The listing builds one solid part. Answer for the finished solid, in the listing's coordinates (mm). Face numbers are marked on the shaded views. A direction names the side the tool comes from. Give positions to 0.01 mm unless a question says otherwise; leave off trailing zeros. Write each loop counter-clockwise with the first axis right and the second up, starting at its lowest first coordinate (ties: lowest second). Pieces come first, ordered by that corner, then holes. Notation, with made-up numbers: M 59,-4.75 L 101,-4.75 A32 cw 101,28.25 Z; hole C 89,35 d10. An arc over 180 degrees is marked long. Return JSON: item names as keys, results as strings.
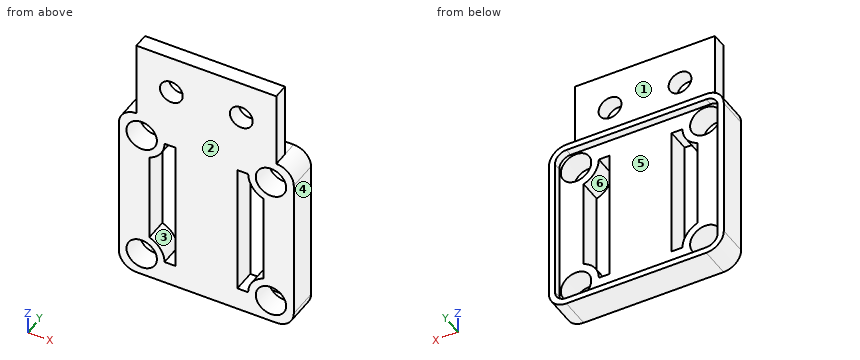
from build123d import *

# Parameters (mm, degrees)
BOSS_EXTRUDE1_DEPTH = 4
CUT_EXTRUDE2_DEPTH  = 1
SKETCH5_R           = 2
CUT_EXTRUDE3_DEPTH  = 22.132971525
CUT_EXTRUDE4_DEPTH  = 22.132971525
SKETCH7_W           = 18.4
SKETCH7_H           = 2
BOSS_EXTRUDE2_DEPTH = 10
SKETCH8_R           = 1.5
CUT_EXTRUDE5_DEPTH  = 25.154392176
CUT_EXTRUDE6_DEPTH  = 1
SKETCH11_W          = 1.421057218
SKETCH11_H          = 17.5
CUT_EXTRUDE7_DEPTH  = 25.257672217


with BuildPart() as part:
    # Sketch1 → Boss-Extrude1 (new body)
    with BuildSketch(Plane(origin=(0, 0, 0), x_dir=(1, 0, 0), z_dir=(0, 1, 0))):
        with BuildLine():
            Line((-12.649074074, 14.633101852), (5.750925926, 14.633101852))
            ThreePointArc((5.750925926, 14.633101852), (7.377271523, 13.959447449), (8.050925926, 12.333101852))
            Line((8.050925926, 12.333101852), (8.050925926, -6.566898148))
            ThreePointArc((8.050925926, -6.566898148), (7.377271523, -8.193243745), (5.750925926, -8.866898148))
            Line((5.750925926, -8.866898148), (-12.649074074, -8.866898148))
            ThreePointArc((-12.649074074, -8.866898148), (-14.275419671, -8.193243745), (-14.949074074, -6.566898148))
            Line((-14.949074074, -6.566898148), (-14.949074074, 12.333101852))
            ThreePointArc((-14.949074074, 12.333101852), (-14.275419671, 13.959447449), (-12.649074074, 14.633101852))
        make_face()
    extrude(amount=BOSS_EXTRUDE1_DEPTH)

    # Sketch2 → Cut-Extrude2 (cut)
    with BuildSketch(Plane(origin=(0, 4, 0), x_dir=(1, 0, 0), z_dir=(0, 1, 0))):
        with BuildLine():
            Line((5.750925926, 13.633101852), (-12.649074074, 13.633101852))
            ThreePointArc((-12.649074074, 13.633101852), (-13.56831289, 13.252340667), (-13.949074074, 12.333101852))
            Line((-13.949074074, 12.333101852), (-13.949074074, -6.566898148))
            ThreePointArc((-13.949074074, -6.566898148), (-13.56831289, -7.486136964), (-12.649074074, -7.866898148))
            Line((-12.649074074, -7.866898148), (5.750925926, -7.866898148))
            ThreePointArc((5.750925926, -7.866898148), (6.670164741, -7.486136964), (7.050925926, -6.566898148))
            Line((7.050925926, -6.566898148), (7.050925926, 12.333101852))
            ThreePointArc((7.050925926, 12.333101852), (6.670164741, 13.252340667), (5.750925926, 13.633101852))
        make_face()
    extrude(amount=-CUT_EXTRUDE2_DEPTH, mode=Mode.SUBTRACT)

    # Sketch5 → Cut-Extrude3 (cut, through all)
    with BuildSketch(Plane(origin=(0, 3, 0), x_dir=(1, 0, 0), z_dir=(0, 1, 0))):
        with Locations(Location((5.050925926, 11.633101852, 0), (0, 0, 270))):
            Circle(SKETCH5_R)
        with Locations(Location((5.050925926, -5.866898148, 0), (0, 0, 270))):
            Circle(SKETCH5_R)
        with Locations(Location((-11.949074074, -5.866898148, 0), (0, 0, 270))):
            Circle(SKETCH5_R)
        with Locations(Location((-11.949074074, 11.633101852, 0), (0, 0, 90))):
            Circle(SKETCH5_R)
    extrude(amount=-CUT_EXTRUDE3_DEPTH, mode=Mode.SUBTRACT)

    # Sketch6 → Cut-Extrude4 (cut, through all)
    with BuildSketch(Plane(origin=(0, 3, 0), x_dir=(1, 0, 0), z_dir=(0, 1, 0))):
        with BuildLine():
            Line((4.050925926, -3.038471023), (4.050925926, 8.804674727))
            ThreePointArc((4.050925926, 8.804674727), (2.601436183, 9.901051044), (2.050925926, 11.633101852))
            Line((2.050925926, 11.633101852), (2.050925926, -5.866898148))
            ThreePointArc((2.050925926, -5.866898148), (2.601436183, -4.134847341), (4.050925926, -3.038471023))
        make_face()
        with BuildLine():
            Line((-10.949074074, 8.804674727), (-10.949074074, -3.038471023))
            ThreePointArc((-10.949074074, -3.038471023), (-9.499584331, -4.134847341), (-8.949074074, -5.866898148))
            Line((-8.949074074, -5.866898148), (-8.949074074, 11.633101852))
            ThreePointArc((-8.949074074, 11.633101852), (-9.499584331, 9.901051044), (-10.949074074, 8.804674727))
        make_face()
    extrude(amount=-CUT_EXTRUDE4_DEPTH, mode=Mode.SUBTRACT)

    # Sketch7 → Boss-Extrude2 (add)
    with BuildSketch(Plane.XY.offset(8.866898148)):
        with Locations((-3.449074074, 1)):
            Rectangle(SKETCH7_W, SKETCH7_H)
    extrude(amount=BOSS_EXTRUDE2_DEPTH)

    # Sketch8 → Cut-Extrude5 (cut, through all)
    with BuildSketch(Plane(origin=(0, 2, 0), x_dir=(1, 0, 0), z_dir=(0, 1, 0))):
        with Locations(Location((1.150925926, -13.866898148, 0), (0, 0, 270))):
            Circle(SKETCH8_R)
        with Locations(Location((-8.049074074, -13.866898148, 0), (0, 0, 270))):
            Circle(SKETCH8_R)
    extrude(amount=-CUT_EXTRUDE5_DEPTH, mode=Mode.SUBTRACT)

    # Sketch9 → Cut-Extrude6 (cut)
    with BuildSketch(Plane(origin=(0, 4, 0), x_dir=(1, 0, 0), z_dir=(0, 1, 0))):
        with BuildLine():
            Line((5.750925926, 13.833101852), (-12.649074074, 13.833101852))
            ThreePointArc((-12.649074074, 13.833101852), (-13.709734246, 13.393762024), (-14.149074074, 12.333101852))
            Line((-14.149074074, 12.333101852), (-14.149074074, -6.566898148))
            ThreePointArc((-14.149074074, -6.566898148), (-13.709734246, -7.62755832), (-12.649074074, -8.066898148))
            Line((-12.649074074, -8.066898148), (5.750925926, -8.066898148))
            ThreePointArc((5.750925926, -8.066898148), (6.811586098, -7.62755832), (7.250925926, -6.566898148))
            Line((7.250925926, -6.566898148), (7.250925926, 12.333101852))
            ThreePointArc((7.250925926, 12.333101852), (6.811586098, 13.393762024), (5.750925926, 13.833101852))
        make_face()
    extrude(amount=-CUT_EXTRUDE6_DEPTH, mode=Mode.SUBTRACT)

    # Sketch11 → Cut-Extrude7 (cut, through all)
    with BuildSketch(Plane(origin=(0, 3, 0), x_dir=(1, 0, 0), z_dir=(0, 1, 0))):
        with Locations((-8.238545465, 2.883101852)):
            Rectangle(SKETCH11_W, SKETCH11_H)
        with Locations((1.340397317, 2.883101852)):
            Rectangle(SKETCH11_W, SKETCH11_H)
    extrude(amount=-CUT_EXTRUDE7_DEPTH, mode=Mode.SUBTRACT)


solid = part.part
Item 1: A cutting plane is placed at B-B, the plane x = -8.5. Write down the section's boundary in (y, z), plus the area to 3 significant figures.
Geometry results:
{"outline": "M 0,-14.63 L 4,-14.63 L 4,-13.83 L 3,-13.83 L 3,-11.63 L 0,-11.63 Z; M 0,5.87 L 3,5.87 L 3,8.07 L 4,8.07 L 4,8.87 L 2,8.87 L 2,12.44 L 0,12.44 Z; M 0,15.3 L 2,15.3 L 2,18.87 L 0,18.87 Z", "area": "33.9 mm2"}
Item 2: Determine the mould class of the marked faces 1, 2 and 3 for opening direction Y: +Y half, -Y half, draft (parallel to the pull), parting line (faces both ways), or undercut.
Geometry results:
{"face 1": "+Y half", "face 2": "-Y half", "face 3": "draft"}
Item 3: Given pin 1 Ø12 at (x, z) = (-4, -11) entering from +Y; pin 2 Ø6.5 at (x, z) = (-0.5, -1.5) entering from +Y; pin 3 Ø8 at (x, z) = (-1, 15.5) entering from +Y; pin 4 Ø1 at (y, z) = (1, 15.5) entering from +X, each flat-ended and moving along its own axis, determine where each tip first touches the part or whether it passes through.
Geometry results:
{"pin 1": "stops at y = 4", "pin 2": "stops at y = 3", "pin 3": "stops at y = 2", "pin 4": "stops at x = 5.75"}
Item 4: A cutting plane is placed at C-C, the plane y = 3.6. Write down the section's boundary in (x, z).
Geometry results:
{"outline": "M -14.95,-12.33 A2.3 ccw -12.65,-14.63 L 5.75,-14.63 A2.3 ccw 8.05,-12.33 L 8.05,6.57 A2.3 ccw 5.75,8.87 L -12.65,8.87 A2.3 ccw -14.95,6.57 Z; hole M -14.15,-12.33 A1.5 ccw -12.65,-13.83 L 5.75,-13.83 A1.5 ccw 7.25,-12.33 L 7.25,6.57 A1.5 ccw 5.75,8.07 L -12.65,8.07 A1.5 ccw -14.15,6.57 Z"}
Item 5: A cutting plane is placed at D-D, the plane y = 1.05. Count the separate pieces of the cut face and the enclosed holes in it, plus the area to 3 significant figures.
Geometry results:
{"separate pieces": "1", "enclosed holes": "8", "area": "552 mm2"}
Item 6: A cutting plane is placed at A-A, the plane z = -6. Write down the section's boundary in (x, y), plus the area to 3 significant figures.
Geometry results:
{"outline": "M -14.95,0 L -10.95,0 L -10.95,3 L -14.15,3 L -14.15,4 L -14.95,4 Z; M -7.53,0 L 0.63,0 L 0.63,3 L -7.53,3 Z; M 4.05,0 L 8.05,0 L 8.05,4 L 7.25,4 L 7.25,3 L 4.05,3 Z", "area": "50.1 mm2"}
Item 7: Find the intervals of material crossed by line 1 (X direction, y = 2.95, z = -7); line 2 (Z direction, x = 2, y = 2.6); line 3 (Z direction, x = 4, y = 1.9), in increasing order.
Geometry results:
{"line 1": "x = -14.95 to -10.95, -7.53 to 0.63, 4.05 to 8.05", "line 2": "z = -14.63 to -11.63, 5.87 to 8.87", "line 3": "z = -14.63 to -13.33, -9.93 to -8.82, 3.06 to 4.17, 7.57 to 18.87"}
Item 8: Which of the six approach directions +Z, -Z, +X, -X, +Y, -Y give full straight-line access (tool end or side, diameter ignored) to the marked faces 4, 5 and 6?
Geometry results:
{"face 4": "+Z, -Z, +X, +Y, -Y", "face 5": "+Y", "face 6": "+Y, -Y"}
